Check sheet for the drawn part. Datum: minimum x, y, z corner. Units: mm. A direction names the side the tool comes from. Round coordinates to 2 decimals unless told otherwise and drop trailing zeros. Write each loop counter-clockwise with the first axis right and the second up, starting at its lowest first coordinate (ties: lowest second). Pieces come first, ordered by that corner, then holes. Notation, with made-up numbers: (3.5, 60.25) -> (45.5, 60.25) arc R22 ccw to (45.5, 81.25) -> close; hole circle Ø8 at (-25, 19.25). An arc over 180 degrees is marked (long way). Use CSV: the item, a comma, the result in double quotes.
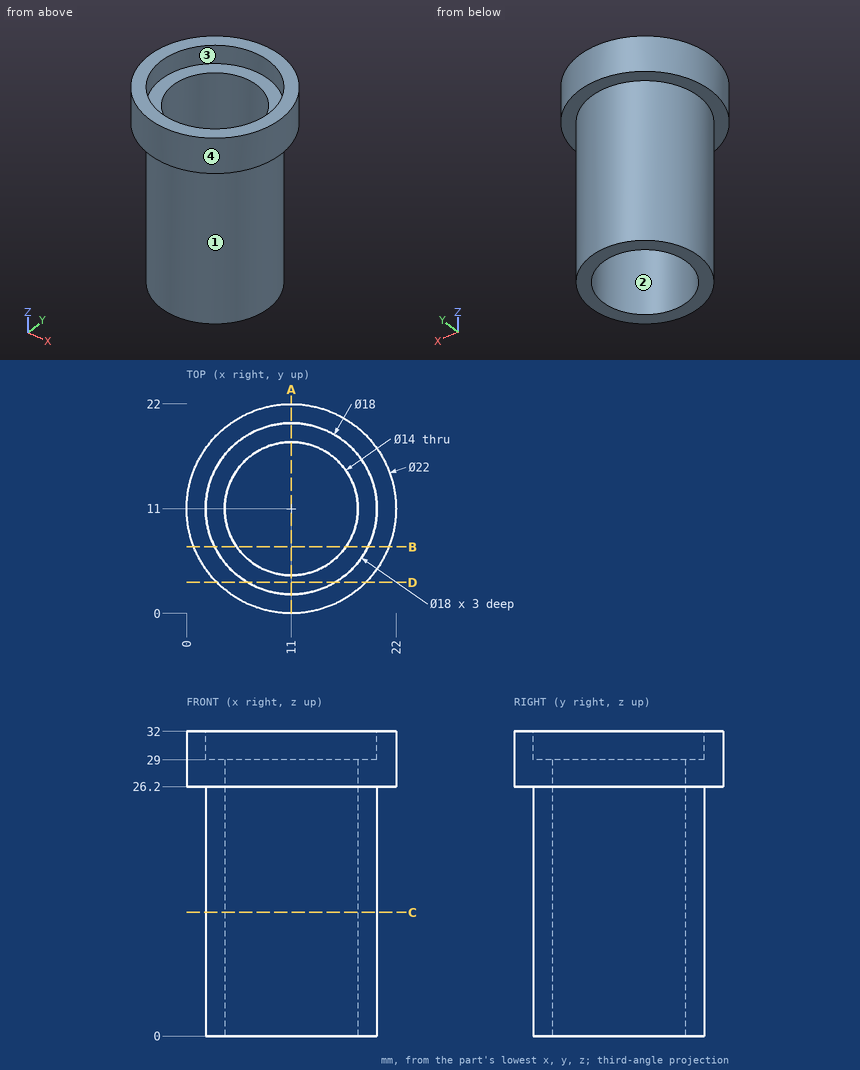
Q1. Section check C-C (z = 13). Record the cut outline in (x, y).
Filled in:
outline,"circle Ø18 at (11, 11); hole circle Ø14 at (11, 11)"
Q2. Material ranges on L1, parallel to Y at x = 11, z = 13; L2, parallel to Y at x = 11, z = 29.75; L3, parallel to Z at x = 18, y = 15.5, recorded low to high.
Filled in:
L1,"2 to 4, 18 to 20"
L2,"0 to 2, 20 to 22"
L3,"0 to 29"
Q3. Go/stop test with flat-tipped pins: P1, Ø10, axis at x = 17.5, z = 14.5, coming from the +Y side; P2, Ø5, axis at y = 13.5, z = 14, coming from the +X side; P3, Ø2, axis at x = 18.5, y = 18.5, coming from the -Z side. Record where each tip stops, or that it passes through.
Filled in:
P1,"y = 19.87"
P2,"x = 20"
P3,"z = 26.2"
Q4. Section check D-D (y = 3.25). Record the cut outline in (x, z), plus the area to 3 significant figures.
Filled in:
outline,"(3.19, 26.2) -> (6.42, 26.2) -> (6.42, 0) -> (15.58, 0) -> (15.58, 26.2) -> (18.81, 26.2) -> (18.81, 32) -> (15.58, 32) -> (15.58, 29) -> (6.42, 29) -> (6.42, 32) -> (3.19, 32) -> close"
area,"303 mm²"
Q5. Section check B-B (y = 7). Record the cut outline in (x, z), plus the area to 3 significant figures.
Filled in:
outline,"(0.75, 26.2) -> (2.94, 26.2) -> (2.94, 0) -> (5.26, 0) -> (5.26, 29) -> (2.94, 29) -> (2.94, 32) -> (0.75, 32) -> close; (16.74, 0) -> (19.06, 0) -> (19.06, 26.2) -> (21.25, 26.2) -> (21.25, 32) -> (19.06, 32) -> (19.06, 29) -> (16.74, 29) -> close"
area,"160 mm²"
Q6. Section check A-A (x = 11). Record the cut outline in (y, z), plus the area to 3 significant figures.
Filled in:
outline,"(0, 26.2) -> (2, 26.2) -> (2, 0) -> (4, 0) -> (4, 29) -> (2, 29) -> (2, 32) -> (0, 32) -> close; (18, 0) -> (20, 0) -> (20, 26.2) -> (22, 26.2) -> (22, 32) -> (20, 32) -> (20, 29) -> (18, 29) -> close"
area,"139 mm²"
Q7. Access from +Z, -Z, +X, -X, +Y, -Y to the whole of each face (thin tool, end or side, straight path). Record for the marked faces 1 and 2.
Filled in:
face 1,"-Z"
face 2,"+Z, -Z"
Q8. Mould release check, pull along X, two halves, no side actions. Record for the marked faces 3 and 4: released by +X, released by -X, zero draft, split by the parting line, or undercut.
Filled in:
face 3,"undercut"
face 4,"split by the parting line"
